Design review of the part built by this model. Coordinates are the model's own, in mm. A direction names the side the tool comes from. Round coordinates to 2 decimals unless told otherwise and drop trailing zeros. Loops run counter-clockwise (first coordinate to the right, second up) from the corner with the lowest first, then second, coordinate; pieces in that order, holes last. Notation, with made-up numbers: (14.5, 32) - (34.5, 32) arc R24 ccw to (34.5, 47) - close; hole circle Ø7 at (-29.5, -38). An arc over 180 degrees is marked (long way). Answer as CSV lines item,"result". Start each with the question number.
(1) Consider section D-D (x = 11). Give the boundary of the cut face in (y, z).
(2) Consider section A-A (z = 1.3). Give the boundary of the cut face in (x, y), and give its area (3 significant figures).
(3) Wall thickness on L1, parallel to Y at x = 0, z = 1.8; L2, parallel to Y at x = 9, z = 1.95; L3, parallel to Y at x = -38.5, z = 2.65: over which ranges is each line inside the solid? List them lowest first.
(4) Consider section C-C (x = 0). Give the boundary of the cut face in (y, z).
(5) For faces 1 (the flat face through (-34.326, -2.606, 1.578)), 2 (the flat face through (26, -8.933, 2)), 3 (the flat face through (-26, 8.933, 2)), 4 (the flat face through (-25, -8.933, 2)), list the 3-axis set-ups (+Z, -Z, +X, -X, +Y, -Y) from which the entire face can be reached by the end or side of a thin tool; tool diameter is ignored.
(6) For P1, Ø1.6, axis at x = 17, z = 2, coming from the +Y side; P2, Ø1.5, axis at x = -1.5, z = 1.5, coming from the -Y side; P3, Ø1.6, axis at x = -24.5, z = 1.5, coming from the -Y side, all flat-tipped, find the tip position at first contact; note any pin that passes through.
(7) Consider section B-B (y = 0). Give the boundary of the cut face in (x, z), and give its area (3 significant figures).
from build123d import *

# Parameters (mm, degrees)
SKETCH_1_R      = 2.95
EXTRUDE_1_DEPTH = 3.2


with BuildPart() as part:
    # Эскиз1 → Бобышка-Вытянуть1 (new body)
    with BuildSketch(Plane.XY):
        with BuildLine():
            Line((-43.083575227, 8.933394968), (-8.012144179, 8.933394968))
            ThreePointArc((-8.012144179, 8.933394968), (0, 12), (8.012144179, 8.933394968))
            Line((8.012144179, 8.933394968), (43.083575227, 8.933394968))
            ThreePointArc((43.083575227, 8.933394968), (44, 0), (43.083575227, -8.933394968))
            Line((43.083575227, -8.933394968), (8.012144179, -8.933394968))
            ThreePointArc((8.012144179, -8.933394968), (0, -12), (-8.012144179, -8.933394968))
            Line((-8.012144179, -8.933394968), (-43.083575227, -8.933394968))
            ThreePointArc((-43.083575227, -8.933394968), (-44, 0), (-43.083575227, 8.933394968))
        make_face()
        Circle(SKETCH_1_R, mode=Mode.SUBTRACT)
        with BuildLine():
            Line((-41.178612038, -3.427717743), (-27.278217848, -1.760672051))
            ThreePointArc((-27.278217848, -1.760672051), (-25.61027786, -3.071387962), (-26.920993771, -4.739327949))
            Line((-26.920993771, -4.739327949), (-40.821387962, -6.406373641))
            ThreePointArc((-40.821387962, -6.406373641), (-42.489327949, -5.09565773), (-41.178612038, -3.427717743))
        make_face(mode=Mode.SUBTRACT)
        with BuildLine():
            Line((40.821387962, -6.406373641), (26.920993771, -4.739327949))
            ThreePointArc((26.920993771, -4.739327949), (25.61027786, -3.071387962), (27.278217848, -1.760672051))
            Line((27.278217848, -1.760672051), (41.178612038, -3.427717743))
            ThreePointArc((41.178612038, -3.427717743), (42.489327949, -5.09565773), (40.821387962, -6.406373641))
        make_face(mode=Mode.SUBTRACT)
    extrude(amount=EXTRUDE_1_DEPTH)


solid = part.part
Determined:
1,outline,"(-8.93, 0) - (8.93, 0) - (8.93, 3.2) - (-8.93, 3.2) - close"
2,outline,"(-43.08, -8.93) - (-8.01, -8.93) arc R12 ccw to (8.01, -8.93) - (43.08, -8.93) arc R44 ccw to (43.08, 8.93) - (8.01, 8.93) arc R12 ccw to (-8.01, 8.93) - (-43.08, 8.93) arc R44 ccw to start; hole (-41.18, -3.43) arc R1.5 ccw to (-40.82, -6.41) - (-26.92, -4.74) arc R1.5 ccw to (-27.28, -1.76) - close; hole circle Ø5.9 at (0, 0); hole (26.92, -4.74) - (40.82, -6.41) arc R1.5 ccw to (41.18, -3.43) - (27.28, -1.76) arc R1.5 ccw to start"
2,area,"1,500 mm^2"
3,L1,"y = -12 to -2.95, 2.95 to 12"
3,L2,"y = -8.93 to 8.93"
3,L3,"y = -8.93 to -6.13, -3.11 to 8.93"
4,outline,"(-12, 0) - (-2.95, 0) - (-2.95, 3.2) - (-12, 3.2) - close; (2.95, 0) - (12, 0) - (12, 3.2) - (2.95, 3.2) - close"
5,face 1,"+Z, -Z"
5,face 2,"+Z, -Z, +X, -Y"
5,face 3,"+Z, -Z, -X, +Y"
5,face 4,"+Z, -Z, -X, -Y"
6,P1,"stops at y = 8.93"
6,P2,"stops at y = -11.98"
6,P3,"stops at y = -8.93"
7,outline,"(-44, 0) - (-2.95, 0) - (-2.95, 3.2) - (-44, 3.2) - close; (2.95, 0) - (44, 0) - (44, 3.2) - (2.95, 3.2) - close"
7,area,"263 mm^2"
